from build123d import *

# Parameters (mm, degrees)
SKETCH_1_R          = 7.5
EXTRUDE_1_DEPTH     = 50
SKETCH_2_W          = 5
SKETCH_2_H          = 5
CUT_EXTRUDE_1_DEPTH = 10
SKETCH_3_W          = 5
SKETCH_3_H          = 5
CUT_EXTRUDE_2_DEPTH = 10


with BuildPart() as part:
    # 草图1 → 凸台-拉伸1 (new body)
    with BuildSketch(Plane(origin=(0, 0, 0), x_dir=(1, 0, 0), z_dir=(0, 1, 0))):
        Circle(SKETCH_1_R)
    extrude(amount=EXTRUDE_1_DEPTH)

    # 草图2 → 切除-拉伸1 (cut)
    with BuildSketch(Plane(origin=(0, 50, 0), x_dir=(1, 0, 0), z_dir=(0, 1, 0))):
        Rectangle(SKETCH_2_W, SKETCH_2_H)
    extrude(amount=-CUT_EXTRUDE_1_DEPTH, mode=Mode.SUBTRACT)

    # 草图3 → 切除-拉伸2 (cut)
    with BuildSketch(Plane.XZ):
        Rectangle(SKETCH_3_W, SKETCH_3_H)
    extrude(amount=-CUT_EXTRUDE_2_DEPTH, mode=Mode.SUBTRACT)

    # 草图4 → 切除-旋转1 (revolve, cut)
    with BuildSketch(Plane(origin=(0, 0, 0), x_dir=(0, 0, -1), z_dir=(1, 0, 0))):
        with BuildLine():
            Line((-7.5, 50), (-7.5, 0))
            ThreePointArc((-7.5, 0), (-4.092291539, 25), (-7.5, 50))
        make_face()
    revolve(axis=Axis((0, 0, 0), (0, 1, 0)), mode=Mode.SUBTRACT)


solid = part.part
Input: part model. Units: mm. Frame: model coordinates. A direction names the side the tool comes from. Give positions to 0.01 mm unless a question says otherwise; leave off trailing zeros. Order: outer loops, then holes, each group sorted by start corner. A loop starts at its lowest first (then second) coordinate and runs counter-clockwise, first axis right, second up. Notation, with made-up numbers: (87, 59.25) - (117, 59.25) arc R22 cw to (117, 86.25) - close; hole circle Ø7 at (65.25, -7). An arc over 180 degrees is marked (long way). Answer as a JSON object with one key per item and string values. Group by question number.
Q1. Set-up query: faces 4 (the face through (3, 50, 0)), 5 (the face through (0, 5, -2.5)), 6 (the face through (0, 40, 0)). Return all of +Z, -Z, +X, -X, +Y, -Y with unobstructed straight access to the full face (end or side cutting, diameter ignored); none if empty.
Q2. Cut plane C-C, the plane y = 41. Output: boundary loops of the cut face in (x, z).
Q3. First-contact query: pin 1 Ø4 at (y, z) = (18, -1.5) entering from -X; pin 2 Ø4 at (y, z) = (41, -6) entering from +X; pin 3 Ø4 at (x, z) = (4, -3.5) entering from -Y; pin 4 Ø5.5 at (y, z) = (6, 0.5) entering from -X. Flat tips, straight axial feed; report the tip coordinate or a pass-through.
Q4. Line query: probe 1 along Y at (x, z) = (-1.25, 0.5); probe 2 along X at (y, z) = (44, -0.5); probe 3 along Z at (x, y) = (1, 12). Output: solid intervals per line, ascending.
Q5. Mould query, pull axis Z, two halves, no side actions, for faces 1 (the face through (3, 0, 0)), 2 (the face through (0, 45, -2.5)), 3 (the face through (0, 5, 2.5)). Classes: pulls with the +Z half, pulls with the -Z half, needs draft (parallel to the pull), parting line crosses it, or undercut.
Q6. Cut plane A-A, the plane y = 7.5. Output: boundary loops of the cut face in (x, z), then the cut area to 3 significant figures.
Q7. Cut plane B-B, the plane y = 28. Output: boundary loops of the cut face in (x, z).
Results:
{
 "1": {"face 4": "+Z, -Z, +X, -X, +Y", "face 5": "-Y", "face 6": "+Y"},
 "2": {"outline": "circle Ø10.95 at (0, 0); hole (-2.5, -2.5) - (2.5, -2.5) - (2.5, 2.5) - (-2.5, 2.5) - close"},
 "3": {"pin 1": "x = -4.48", "pin 2": "x = 3.8", "pin 3": "y = 0", "pin 4": "x = -6.65"},
 "4": {"probe 1": "10 to 40", "probe 2": "-6.02 to -2.5, 2.5 to 6.02", "probe 3": "-4.9 to 4.9"},
 "5": {"face 1": "needs draft", "face 2": "undercut", "face 3": "undercut"},
 "6": {"outline": "circle Ø11.49 at (0, 0); hole (-2.5, -2.5) - (2.5, -2.5) - (2.5, 2.5) - (-2.5, 2.5) - close", "area": "78.7 mm^2"},
 "7": {"outline": "circle Ø8.28 at (0, 0)"}
}
